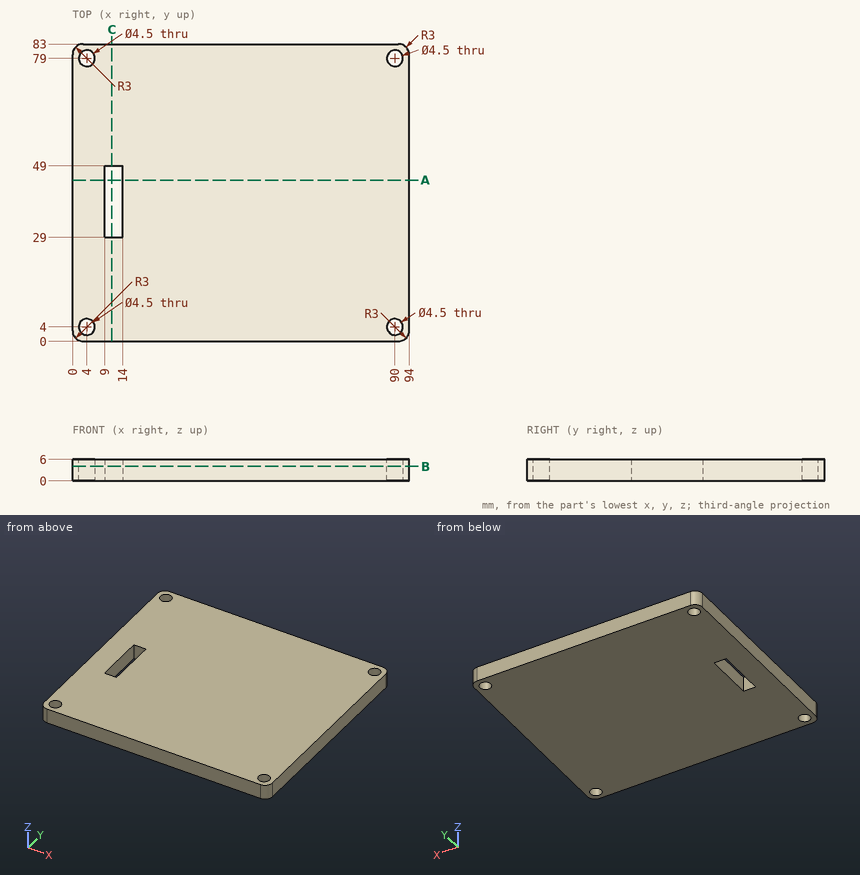
Geometry: see drawing. Coordinates: mm, zero at the bounding-box minimum. Coordinates: 2 decimals unless noted, no trailing zeros. Order: outer loops, then holes, each group sorted by start corner. A loop starts at its lowest first (then second) coordinate and runs counter-clockwise, first axis right, second up. Notation, with made-up numbers: M 66.25,5 L 77.25,5 A12 cw 77.25,23 Z; hole C 21.5,-33 d2. An arc over 180 degrees is marked long. Answer in a Markdown table with one row per item. Add a question column.
Q1. Section query A-A on y = 45. Return the cut outline in (x, z).
Q2. Section query B-B on z = 4.05. Return the cut outline in (x, y), and give its area (3 significant figures).
Q3. Line query: L1, parallel to Y at x = 90, z = 3.9; L2, parallel to X at y = 48, z = 1.95; L3, parallel to Y at x = 88, z = 0.8. Output: solid intervals per line, ascending.
Q4. Contact query for a flat-ended pin moving along its axis: P1, Ø3.5, axis at x = 4, y = 79, coming from the +Z side. Output: stop coordinate, or through.
Q5. Section query C-C on x = 11. Return the cut outline in (y, z), and give its area (3 significant figures).
Completed:
| question | item | result |
|---|---|---|
| 1 | outline | M 0,0 L 9,0 L 9,6 L 0,6 Z; M 14,0 L 94,0 L 94,6 L 14,6 Z |
| 2 | outline | M 0,3 A3 ccw 3,0 L 91,0 A3 ccw 94,3 L 94,80 A3 ccw 91,83 L 3,83 A3 ccw 0,80 Z; hole C 4,4 d4.5; hole C 4,79 d4.5; hole M 9,29 L 14,29 L 14,49 L 9,49 Z; hole C 90,4 d4.5; hole C 90,79 d4.5 |
| 2 | area | 7,630 mm2 |
| 3 | L1 | y = 0 to 1.75, 6.25 to 76.75, 81.25 to 83 |
| 3 | L2 | x = 0 to 9, 14 to 94 |
| 3 | L3 | y = 0 to 2.97, 5.03 to 77.97, 80.03 to 83 |
| 4 | P1 | passes through |
| 5 | outline | M 0,0 L 29,0 L 29,6 L 0,6 Z; M 49,0 L 83,0 L 83,6 L 49,6 Z |
| 5 | area | 378 mm2 |
